from build123d import *

# Parameters (mm, degrees)
F0_R     = 16
F1_DEPTH = 2
F2_R     = 6
F3_DEPTH = 25
F4_W     = 41.035842
F4_H     = 41.410806
F5_DEPTH = 25


with BuildPart() as f1:
    # F0 (on Top) → F1 (new body)
    with BuildSketch(Plane.XY):
        Circle(F0_R)
    extrude(amount=F1_DEPTH)

    # F2 (on Top) → F3 (cut)
    with BuildSketch(Plane.XY):
        Circle(F2_R)
    extrude(amount=F3_DEPTH, mode=Mode.SUBTRACT)

    # F4 (on Top) → F5 (cut)
    with BuildSketch(Plane.XY):
        with Locations((20.517921, 0.114485)):
            Rectangle(F4_W, F4_H)
    extrude(amount=F5_DEPTH, mode=Mode.SUBTRACT)


solid = f1.part
Build history of the part. All positions in model axes, mm. Round coordinates to 2 decimals unless told otherwise and drop trailing zeros. Write each loop counter-clockwise with the first axis right and the second up, starting at its lowest first coordinate (ties: lowest second). Pieces come first, ordered by that corner, then holes. Notation, with made-up numbers: M 21.5,41 L 52.5,41 A37 ccw 52.5,78 Z; hole C 15,-28.5 d9. An arc over 180 degrees is marked long. Use CSV: the item, a comma, the result in double quotes.
1. Saw through at B-B (z = 0.75). Give the cut face in (x, y).
Reply:
outline,"M 0,-16 L 0,-6 A6 cw 0,6 L 0,16 A16 ccw Z"
2. Flat gauge pin, fed straight in: pin 1 (1 mm diameter, centred on x = -10, z = 0.5, fed in from +Y). Where does the tip first touch, or does it go through?
Reply:
pin 1,"stops at y = 12.87"
3. Saw through at A-A (x = -3.5). Give the cut face in (y, z), plus the area to 3 significant figures.
Reply:
outline,"M -15.61,0 L -4.87,0 L -4.87,2 L -15.61,2 Z; M 4.87,0 L 15.61,0 L 15.61,2 L 4.87,2 Z"
area,"43.0 mm²"
4. Saw through at C-C (y = 0). Give the cut face in (x, z).
Reply:
outline,"M -16,0 L -6,0 L -6,2 L -16,2 Z"
5. Wall check: probe 1 along Y at (x, z) = (-2.25, 1.65); probe 2 along Y at (x, z) = (-5, 0.7); probe 3 along Y at (x, z) = (-10.25, 1.4). Give the ranges that are in metal, low to high. Write a range as from..to.
Reply:
probe 1,"y = -15.84..-5.56, 5.56..15.84"
probe 2,"y = -15.2..-3.32, 3.32..15.2"
probe 3,"y = -12.29..12.29"
6. Two-plate mould, pull along Y, no slides. Class faces 1 (the face through (-6, 0, 1)), 2 (the face through (0, 11, 1)), 3 (the face through (-16, 0, 1)): +Y half, -Y half, draft (parallel to the pull), parting line (faces both ways), or undercut.
Reply:
face 1,"undercut"
face 2,"draft"
face 3,"parting line"
